Part model, mm, in its own coordinate system. A direction names the side the tool comes from. Give positions to 0.01 mm unless a question says otherwise; leave off trailing zeros. Order: outer loops, then holes, each group sorted by start corner. A loop starts at its lowest first (then second) coordinate and runs counter-clockwise, first axis right, second up. Notation, with made-up numbers: (31.5, -34) -> (41.5, -34) arc R32 ccw to (41.5, -6) -> close; hole circle Ø9 at (-19, 12.25). An arc over 180 degrees is marked (long way). Write item = value, one per line. Start each with the question number.
Item 1: Drill centre lines: line 1 along X through (y, z) = (0, -4.5); line 2 along Y through (x, z) = (-1.5, -4); line 3 along Z through (x, y) = (1.5, -4.75). Where is each one in solid material? Low to high.
Item 2: Flat gauge pins, fed straight in: P1, Ø4, axis at x = 3.5, z = -6, coming from the +Y side; P2, Ø5, axis at x = 0, y = 0, coming from the +Z side; P3, Ø1.5, axis at y = -1.5, z = -7, coming from the -X side; P4, Ø1.5, axis at y = -4, z = -4.5, coming from the +X side. Where does each tip first touch, or does it go through?
Item 3: Band-saw the part on C-C on z = -1. Write the cut outline in (x, y).
Item 4: Band-saw the part on D-D on z = -4.25. Write the cut outline in (x, y).
Item 5: Pull direction X, two halves, no side cores. Call faces 1 (the face through (-0.9, -2.86, -3.95)), 2 (the face through (-3.1, 1.4, -8)), 3 (the face through (5.37, 1.19, -1.01)): +X half, -X half, draft (parallel to the pull), parting line (faces both ways), or undercut.
Item 6: Band-saw the part on A-A on y = 0. Write the cut outline in (x, z), plus the area to 3 significant figures.
Item 7: Tool access for faces 4 (the face through (2, 4, -2)), 5 (the face through (3.4, -0.1, 0)): list every direction of +Z, -Z, +X, -X, +Y, -Y with a clear straight run to the whole face (end or side of a thin tool).
```python
from build123d import *

# Parameters (mm, degrees)
CHAMFER1_SIZE = 0.25


with BuildPart() as part:
    # Sketch1 → Revolve1 (revolve)
    with BuildSketch(Plane(origin=(0, 0, 0), x_dir=(0, 0, -1), z_dir=(1, 0, 0)), mode=Mode.PRIVATE) as revolve1_sk:
        Polygon((0, 3), (0, 5.5), (2, 5.5), (2, 4), (8, 4), (8, 3), align=None)
    revolve(revolve1_sk.sketch.rotate(Axis((0, 0, 0), (0, 0, -1)), 180), axis=Axis((0, 0, 0), (0, 0, -1)))  # turned: the seam where the file's is

    # Chamfer1
    chamfer1_edges = [part.edges().sort_by_distance(p)[0] for p in [
        (0, 3, -8),
        (0, 4, -8),
        (0, 5.5, -2),
        (0, 5.5, 0),
        (0, 3, 0),
    ]]
    chamfer(chamfer1_edges, length=CHAMFER1_SIZE)


solid = part.part
```
Values found:
q1.line_1 = -4 to -3, 3 to 4
q1.line_2 = -3.71 to -2.6, 2.6 to 3.71
q1.line_3 = -2 to 0
q2.P1 = 3.71
q2.P2 = through
q2.P3 = -3.93
q2.P4 = 2.33
q3.outline = circle Ø11 at (0, 0); hole circle Ø6 at (0, 0)
q4.outline = circle Ø8 at (0, 0); hole circle Ø6 at (0, 0)
q5.face_1 = undercut
q5.face_2 = draft
q5.face_3 = parting line
q6.outline = (-5.5, -1.75) -> (-5.25, -2) -> (-4, -2) -> (-4, -7.75) -> (-3.75, -8) -> (-3.25, -8) -> (-3, -7.75) -> (-3, -0.25) -> (-3.25, 0) -> (-5.25, 0) -> (-5.5, -0.25) -> close; (3, -7.75) -> (3.25, -8) -> (3.75, -8) -> (4, -7.75) -> (4, -2) -> (5.25, -2) -> (5.5, -1.75) -> (5.5, -0.25) -> (5.25, 0) -> (3.25, 0) -> (3, -0.25) -> close
q6.area = 21.7 mm^2
q7.face_4 = -Z
q7.face_5 = +Z, +X, -X, +Y, -Y
